from build123d import *

# Parameters (mm, degrees)
SKETCH1_W               = 55.88
SKETCH1_H               = 83.566
BOSS_EXTRUDE1_DEPTH     = 3.175
SKETCH2_W               = 74.93
SKETCH2_H               = 102.616
SKETCH2_W_2             = 55.88
SKETCH2_H_2             = 83.566
BOSS_EXTRUDE2_DEPTH     = 12.065
CUT_EXTRUDE1_DEPTH      = 65.666075449
CUT_EXTRUDE1_DEPTH_BACK = 65.666075449
SKETCH3_R               = 3.556
CUT_EXTRUDE2_DEPTH      = 65.666075449
CUT_EXTRUDE2_DEPTH_BACK = 65.666075449
SKETCH4_W               = 1.778
SKETCH4_H               = 74.93
FILLET1_R               = 6.35
FILLET2_R               = 0.508
SKETCH5_W               = 38.1
SKETCH5_H               = 3.175
BOSS_EXTRUDE3_DEPTH     = 30.48
CUT_EXTRUDE3_DEPTH      = 89.793346738
CUT_EXTRUDE3_DEPTH_BACK = 89.793346738
SKETCH6_W               = 7.62
SKETCH6_H               = 22.86
SKETCH7_R               = 1.7145
BOSS_EXTRUDE4_DEPTH     = 3.81
CUT_EXTRUDE4_DEPTH      = 89.793346738
CUT_EXTRUDE4_DEPTH_BACK = 89.793346738
SKETCH8_W               = 22.86
SKETCH8_H               = 15.875
SKETCH9_W               = 6.6929
SKETCH9_H               = 15.875
BOSS_EXTRUDE5_DEPTH     = 3.175
FILLET3_R               = 19.05
FILLET5_R               = 1.27
SKETCH14_W              = 22.86
SKETCH14_H              = 3.175
BOSS_EXTRUDE8_DEPTH     = 12.7
CUT_EXTRUDE7_DEPTH      = 95.853357479
CUT_EXTRUDE7_DEPTH_BACK = 95.853357479
CUT_EXTRUDE8_DEPTH      = 95.853357479
CUT_EXTRUDE8_DEPTH_BACK = 95.853357479
SKETCH16_W              = 17.130818864
SKETCH16_H              = 3.4036
FILLET8_R               = 0.508
SKETCH17_R              = 0.889
BOSS_EXTRUDE9_DEPTH     = 2.54


with BuildPart() as part:
    # Sketch1 → Boss-Extrude1 (new body)
    with BuildSketch(Plane(origin=(0, 0, 0), x_dir=(0, 1, 0), z_dir=(0, 0, 1))):
        Rectangle(SKETCH1_W, SKETCH1_H)
    extrude(amount=BOSS_EXTRUDE1_DEPTH)

    # Sketch2 → Boss-Extrude2 (add)
    with BuildSketch(Plane(origin=(0, 0, 0), x_dir=(0, 1, 0), z_dir=(0, 0, 1))):
        Rectangle(SKETCH2_W, SKETCH2_H)
        Rectangle(SKETCH2_W_2, SKETCH2_H_2, mode=Mode.SUBTRACT)
    extrude(amount=BOSS_EXTRUDE2_DEPTH)

    # Sketch3 → Cut-Extrude1 (cut, two sides: drawn at the far end of the back side and taken through both)
    with BuildSketch(Plane.XY.offset(12.065).offset(-CUT_EXTRUDE1_DEPTH_BACK)):
        with Locations((-43.815, 31.75)):
            Circle(SKETCH3_R)
        with Locations((43.815, 31.75)):
            Circle(SKETCH3_R)
        with Locations((43.815, -31.75)):
            Circle(SKETCH3_R)
        with Locations((-43.815, -31.75)):
            Circle(SKETCH3_R)
    extrude(amount=CUT_EXTRUDE1_DEPTH + CUT_EXTRUDE1_DEPTH_BACK, mode=Mode.SUBTRACT)

    # Sketch4 → Cut-Extrude2 (cut, two sides: drawn at the far end of the back side and taken through both)
    with BuildSketch(Plane.XY.offset(12.065).offset(-CUT_EXTRUDE2_DEPTH_BACK)):
        with Locations((-50.419, 0)):
            Rectangle(SKETCH4_W, SKETCH4_H)
        with Locations((50.419, 0)):
            Rectangle(SKETCH4_W, SKETCH4_H)
    extrude(amount=CUT_EXTRUDE2_DEPTH + CUT_EXTRUDE2_DEPTH_BACK, mode=Mode.SUBTRACT)

    # Fillet1
    fillet1_edges = [part.edges().sort_by_distance(p)[0] for p in [
        (-49.53, -37.465, 6.0325),
        (-49.53, 37.465, 6.0325),
        (49.53, 37.465, 6.0325),
        (49.53, -37.465, 6.0325),
    ]]
    fillet(fillet1_edges, radius=FILLET1_R)

    # Fillet2
    fillet2_edges = [part.edges().sort_by_distance(p)[0] for p in [
        (-47.371, -31.75, 0),
        (40.259, -31.75, 0),
        (40.259, 31.75, 0),
        (-47.371, 31.75, 0),
    ]]
    fillet(fillet2_edges, radius=FILLET2_R)

    # Sketch5 → Boss-Extrude3 (add)
    with BuildSketch(Plane.YZ.offset(49.53)):
        with Locations((0, 1.5875)):
            Rectangle(SKETCH5_W, SKETCH5_H)
    extrude(amount=BOSS_EXTRUDE3_DEPTH)

    # Sketch6 → Cut-Extrude3 (cut, two sides: drawn at the far end of the back side and taken through both)
    with BuildSketch(Plane.XY.offset(3.175).offset(-CUT_EXTRUDE3_DEPTH_BACK)):
        with Locations((53.34, 0)):
            Rectangle(SKETCH6_W, SKETCH6_H)
    extrude(amount=CUT_EXTRUDE3_DEPTH + CUT_EXTRUDE3_DEPTH_BACK, mode=Mode.SUBTRACT)

    # Sketch7 → Boss-Extrude4 (add)
    with BuildSketch(Plane.XY.offset(3.175)):
        with Locations(Location((53.3019, 13.9573, 0), (0, 0, 180))):
            Circle(SKETCH7_R)
        with Locations(Location((53.3019, -13.9573, 0), (0, 0, 180))):
            Circle(SKETCH7_R)
    extrude(amount=BOSS_EXTRUDE4_DEPTH)

    # Sketch8 → Cut-Extrude4 (cut, two sides: drawn at the far end of the back side and taken through both)
    with BuildSketch(Plane.XY.offset(3.175).offset(-CUT_EXTRUDE4_DEPTH_BACK)):
        with Locations((68.58, 0)):
            Rectangle(SKETCH8_W, SKETCH8_H)
    extrude(amount=CUT_EXTRUDE4_DEPTH + CUT_EXTRUDE4_DEPTH_BACK, mode=Mode.SUBTRACT)

    # Sketch9 → Boss-Extrude5 (add)
    with BuildSketch(Plane.XY.offset(3.175)):
        with Locations((76.66355, 0)):
            Rectangle(SKETCH9_W, SKETCH9_H)
    extrude(amount=-BOSS_EXTRUDE5_DEPTH)

    # Fillet3
    fillet3_edges = [part.edges().sort_by_distance(p)[0] for p in [
        (80.01, -19.05, 1.5875),
        (80.01, 19.05, 1.5875),
    ]]
    fillet(fillet3_edges, radius=FILLET3_R - 0.0001)  # a hair under: the kernel refuses the full size

    # Fillet5
    fillet5_edges = [part.edges().sort_by_distance(p)[0] for p in [
        (57.15, 11.43, 1.5875),
        (57.15, -11.43, 1.5875),
        (57.15, 7.9375, 1.5875),
        (57.15, -7.9375, 1.5875),
    ]]
    fillet(fillet5_edges, radius=FILLET5_R)

    # Sketch14 → Boss-Extrude8 (add)
    with BuildSketch(Plane(origin=(0, 37.465, 0), x_dir=(-1, 0, 0), z_dir=(0, 1, 0))):
        with Locations((0, 1.5875)):
            Rectangle(SKETCH14_W, SKETCH14_H)
    extrude(amount=BOSS_EXTRUDE8_DEPTH)

    # Sketch15 → Cut-Extrude7 (cut, two sides: drawn at the far end of the back side and taken through both)
    with BuildSketch(Plane.XY.offset(3.175).offset(-CUT_EXTRUDE7_DEPTH_BACK)):
        with BuildLine():
            Line((-1.905, 49.276), (1.905, 49.276))
            ThreePointArc((1.905, 49.276), (6.35, 44.831), (1.905, 40.386))
            Line((1.905, 40.386), (-1.905, 40.386))
            ThreePointArc((-1.905, 40.386), (-6.35, 44.831), (-1.905, 49.276))
        make_face()
    extrude(amount=CUT_EXTRUDE7_DEPTH + CUT_EXTRUDE7_DEPTH_BACK, mode=Mode.SUBTRACT)

    # Sketch16 → Cut-Extrude8 (cut, two sides: drawn at the far end of the back side and taken through both)
    with BuildSketch(Plane.XY.offset(3.175).offset(-CUT_EXTRUDE8_DEPTH_BACK)):
        with Locations((0, 39.1668)):
            Rectangle(SKETCH16_W, SKETCH16_H)
    extrude(amount=CUT_EXTRUDE8_DEPTH + CUT_EXTRUDE8_DEPTH_BACK, mode=Mode.SUBTRACT)

    # Fillet8
    fillet8_edges = [part.edges().sort_by_distance(p)[0] for p in [
        (3.919301676, 40.8686, 1.5875),
        (-3.919301676, 40.8686, 1.5875),
    ]]
    fillet(fillet8_edges, radius=FILLET8_R)

    # Sketch17 → Boss-Extrude9 (add)
    with BuildSketch(Plane.XY.offset(3.175)):
        with Locations((-7.8994, 44.577)):
            Circle(SKETCH17_R)
        with Locations((7.8994, 44.577)):
            Circle(SKETCH17_R)
    extrude(amount=BOSS_EXTRUDE9_DEPTH)


solid = part.part
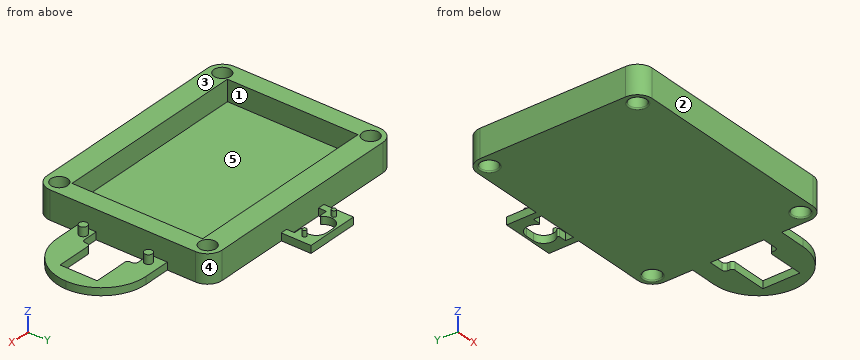
The listing builds one solid part. Answer for the finished solid, in the listing's coordinates (mm). Face numbers are marked on the shaded views. A direction names the side the tool comes from. Coordinates: 2 decimals unless noted, no trailing zeros. Write each loop counter-clockwise with the first axis right and the second up, starting at its lowest first coordinate (ties: lowest second). Pieces come first, ordered by that corner, then holes. Notation, with made-up numbers: (22.25, 45.5) -> (48.25, 45.5) arc R15 ccw to (48.25, 56.5) -> close; hole circle Ø7 at (40, 48). An arc over 180 degrees is marked (long way). One line per question, with ' | ' between items.
1. Straight lines are drawn through the part: line 1 (Y direction, x = 34.5, z = 9) (3 decimals); line 2 (X direction, y = 3, z = 9.25); line 3 (X direction, y = 31.75, z = 6). For each, find the intervals that lie inside material, in ascending order.
Verdict:
line 1: y = -37.465 to -27.94, 27.94 to 37.465 | line 2: x = -49.53 to -41.78, 41.78 to 49.53 | line 3: x = -49.5 to -47.37, -40.26 to 40.26, 47.37 to 49.5
2. Section C-C (y = 25) is taken. Determine the outline of the cut face in (x, z) (3 decimals).
Verdict:
outline: (-49.53, 0) -> (49.53, 0) -> (49.53, 12.065) -> (41.783, 12.065) -> (41.783, 3.175) -> (-41.783, 3.175) -> (-41.783, 12.065) -> (-49.53, 12.065) -> close
3. Given pin 1 Ø5 at (y, z) = (4, 5) entering from +X; pin 2 Ø8 at (x, y) = (-43.815, -31.75) entering from -Z; pin 3 Ø3 at (x, z) = (28.5, 1.5) entering from +Y (3 decimals), each flat-ended and moving along its own axis, determine where each tip first touches the part or whether it passes through.
Verdict:
pin 1: stops at x = 79.87 | pin 2: stops at z = 0 | pin 3: stops at y = 37.465
4. Section B-B (x = 70) is taken. Determine the outline of the cut face in (y, z) (1 decimal).
Verdict:
outline: (-16.8, 0) -> (-7.9, 0) -> (-7.9, 3.2) -> (-16.8, 3.2) -> close; (7.9, 0) -> (16.8, 0) -> (16.8, 3.2) -> (7.9, 3.2) -> close
5. Section D-D (y = 4) is taken. Determine the outline of the cut face in (x, z) (3 decimals).
Verdict:
outline: (-49.53, 0) -> (49.53, 0) -> (49.53, 12.065) -> (41.783, 12.065) -> (41.783, 3.175) -> (-41.783, 3.175) -> (-41.783, 12.065) -> (-49.53, 12.065) -> close; (73.317, 0) -> (79.585, 0) -> (79.585, 3.175) -> (73.317, 3.175) -> close
6. Section A-A (z = 9.75) is taken. Determine the outline of the cut face in (x, y) (3 decimals), and give its area (3 significant figures).
Verdict:
outline: (-49.53, -31.115) arc R6.35 ccw to (-43.18, -37.465) -> (43.18, -37.465) arc R6.35 ccw to (49.53, -31.115) -> (49.53, 31.115) arc R6.35 ccw to (43.18, 37.465) -> (-43.18, 37.465) arc R6.35 ccw to (-49.53, 31.115) -> close; hole circle Ø7.112 at (-43.815, -31.75); hole circle Ø7.112 at (-43.815, 31.75); hole (-41.783, -27.94) -> (41.783, -27.94) -> (41.783, 27.94) -> (-41.783, 27.94) -> close; hole circle Ø7.112 at (43.815, -31.75); hole circle Ø7.112 at (43.815, 31.75) | area: 2,560 mm^2
7. For a pull along Y with two mould halves and no side action, classify the marked faces 1, 2 and 3 as released by +Y, released by -Y, zero draft, split by the parting line, or undercut.
Verdict:
face 1: undercut | face 2: released by -Y | face 3: zero draft
8. Which of the six approach directions +Z, -Z, +X, -X, +Y, -Y give full straight-line access (tool end or side, diameter ignored) to the marked faces 4 and 5?
Verdict:
face 4: +Z, -Z, +X, +Y | face 5: +Z
